from build123d import *

# Parameters (mm, degrees)
F2_R      = 139.7
F3_DEPTH  = 19.05
F4_SIZE   = 1.5875
F5_R      = 120.65
F6_DEPTH  = 19.051
F7_W      = 12.7
F7_H      = 5.55625
F8_DEPTH  = 139.701
F9_R      = 0.79375
F10_DEPTH = 19.051


# Not quite as in the source:
# - a variable given as a bare number and used for a length is read in inches; the dataset says mm whatever the document's units were


with BuildPart() as f3:
    # F2 (on Top) → F3 (new body)
    with BuildSketch(Plane.XY):
        Circle(F2_R)
    extrude(amount=F3_DEPTH)

    # F4
    f4_edges = [f3.edges().sort_by_distance(p)[0] for p in [
        (-139.7, 0, 19.05),
        (-139.7, 0, 0),
    ]]
    chamfer(f4_edges, length=F4_SIZE)

    # F5 (on face) → F6 (cut, through all)
    with BuildSketch(Plane(origin=(0, 0, 0), x_dir=(1, 0, 0), z_dir=(0, 0, -1))):
        Circle(F5_R)
    extrude(amount=-F6_DEPTH, mode=Mode.SUBTRACT)

    # F7 (on Front) → F8 (cut, through all)
    with BuildSketch(Plane.XZ):
        with Locations((0, 2.778125)):
            Rectangle(F7_W, F7_H)
    extrude(amount=F8_DEPTH, mode=Mode.SUBTRACT)

    # F9 (on Top) → F10 (cut, through all)
    with BuildSketch(Plane.XY):
        with Locations((92.047625241, -92.047625241)):
            Circle(F9_R)
        with Locations((-92.047625241, -92.047625241)):
            Circle(F9_R)
        with Locations((-92.047625241, 92.047625241)):
            Circle(F9_R)
        with Locations((92.047625241, 92.047625241)):
            Circle(F9_R)
    extrude(amount=F10_DEPTH, mode=Mode.SUBTRACT)


solid = f3.part
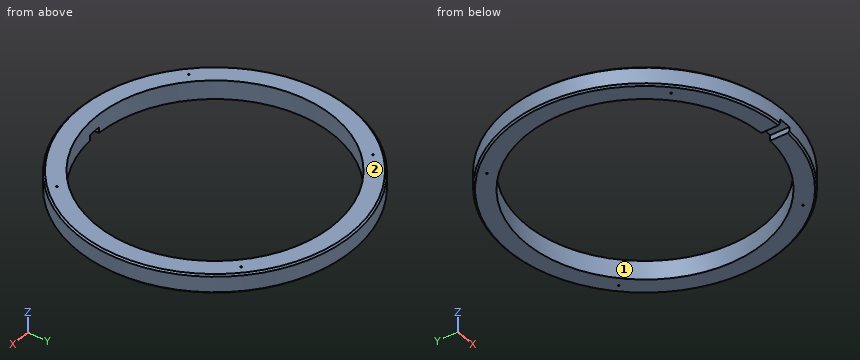
Design review of the part built by this model. Coordinates are the model's own, in mm. Face numbers are marked on the shaded views. Give positions to 0.01 mm unless a question says otherwise; leave off trailing zeros. Order: outer loops, then holes, each group sorted by start corner. A loop starts at its lowest first (then second) coordinate and runs counter-clockwise, first axis right, second up.
1. To check wall thickness, follow L1, parallel to Y at x = -2, z = 7; L2, parallel to X at y = 2.5, z = 10.75; L3, parallel to X at y = 95, z = 17.75. State the ranges of each line that lie inside material, in increasing order.
Solution:
L1: y = -139.69 to -120.63, 120.63 to 139.69
L2: x = -139.68 to -120.62, 120.62 to 139.68
L3: x = -102.03 to -74.37, 74.37 to 102.03
2. Mouldability with a two-part tool opening along Y and no side actions: class the marked faces 1 and 2 as +Y half, -Y half, draft (parallel to the pull), parting line (faces both ways), or undercut.
Solution:
face 1: undercut
face 2: draft
3. For pin 1 Ø5 at (x, z) = (42, 3.5) entering from -Y; pin 2 Ø6 at (y, z) = (-126, 4) entering from -X; pin 3 Ø8 at (x, z) = (-9.5, 12) entering from -Y, all flat-tipped, find the tip position at first contact; note any pin that passes through.
Solution:
pin 1: stops at y = -134
pin 2: stops at x = -66.24
pin 3: stops at y = -139.59
4. Add section B-B, the plane z = 8.75. State the section outline as (x, y) points.
Solution:
outline: circle Ø279.4 at (0, 0); hole circle Ø241.3 at (0, 0); hole circle Ø1.59 at (-92.05, -92.05); hole circle Ø1.59 at (-92.05, 92.05); hole circle Ø1.59 at (92.05, -92.05); hole circle Ø1.59 at (92.05, 92.05)
5. Add section A-A, the plane x = 0. State the section outline as (y, z) points, then the cut area to 3 significant figures.
Solution:
outline: (-139.7, 5.56) - (-120.65, 5.56) - (-120.65, 19.05) - (-138.11, 19.05) - (-139.7, 17.46) - close; (120.65, 0) - (138.11, 0) - (139.7, 1.59) - (139.7, 17.46) - (138.11, 19.05) - (120.65, 19.05) - close
area: 616 mm2
